Here's how the part is built. I have some questions about the finished solid (model axes, mm). A direction names the side the tool comes from. Give positions to 0.01 mm unless a question says otherwise; leave off trailing zeros. Loops run counter-clockwise (first coordinate to the right, second up) from the corner with the lowest first, then second, coordinate; pieces in that order, holes last. Notation, with made-up numbers: (-24, 22) - (-20, 22) arc R21 cw to (-20, 41) - close; hole circle Ø4 at (58.25, 12). An arc over 180 degrees is marked (long way). Use one line per item in the form item = value.
from build123d import *

# Parameters (mm, degrees)
F0_R     = 3.175
F1_DEPTH = 3.175


with BuildPart() as f1:
    # F0 (on Right) → F1 (new body)
    with BuildSketch(Plane.YZ):
        with BuildLine():
            Line((-11.176, 44.45), (-7.62, 0))
            ThreePointArc((-7.62, 0), (0, -7.62), (7.62, 0))
            Line((7.62, 0), (9.542272, 24.0284))
            ThreePointArc((9.542272, 24.0284), (11.848513, 29.596159), (17.416272, 31.9024))
            Line((17.416272, 31.9024), (63.5, 27.810218))
            Line((63.5, 27.810218), (115.700079, 31.9024))
            ThreePointArc((115.700079, 31.9024), (125.810106, 43.319551), (115.700079, 54.736701))
            Line((115.700079, 54.736701), (63.5, 61.099302))
            Line((63.5, 61.099302), (0, 55.626))
            ThreePointArc((0, 55.626), (-7.902625, 52.352625), (-11.176, 44.45))
        make_face()
        Circle(F0_R, mode=Mode.SUBTRACT)
        with Locations((0, 44.45)):
            Circle(F0_R, mode=Mode.SUBTRACT)
        with Locations((63.5, 44.45)):
            Circle(F0_R, mode=Mode.SUBTRACT)
        with Locations((99.822, 47.625)):
            Circle(F0_R, mode=Mode.SUBTRACT)
        with Locations((114.3, 44.45)):
            Circle(F0_R, mode=Mode.SUBTRACT)
    extrude(amount=F1_DEPTH)


solid = f1.part
(1) If we section it at D-D (y = 59): List the corners of the cut face in (x, z) for me (3 decimals).
Geometry says:
outline = (0, 28.21) - (3.175, 28.21) - (3.175, 60.711) - (0, 60.711) - close
(2) If we section it at A-A (y = 114.3): List the corners of the cut face in (x, z) for me (3 decimals), plus the area to 3 significant figures.
Geometry says:
outline = (0, 31.793) - (3.175, 31.793) - (3.175, 41.275) - (0, 41.275) - close; (0, 47.625) - (3.175, 47.625) - (3.175, 54.907) - (0, 54.907) - close
area = 53.2 mm²
(3) If I drill on probe 1 along Z at (x, y) = (1.1, 0) (3 decimals); probe 2 along Z at (x, y) = (2.7, 1.5); probe 3 along Y at (x, z) = (0.45, 48), over which ranges is the centre line in solid material (lowest first)?
Geometry says:
probe_1 = -7.62 to -3.175, 3.175 to 41.275, 47.625 to 55.626
probe_2 = -7.47 to -2.8, 2.8 to 41.65, 47.25 to 55.76
probe_3 = -10.6 to 96.67, 102.97 to 124.81
(4) For faces 1 (the flat face through (1.565, 40.136, 29.885)), 2 (the cylindrical face through (1.565, 1.707, 47.127)), which set-ups out of +Z, -Z, +X, -X, +Y, -Y let a thin tool reach every point of the face, with its end or its side?
Geometry says:
face_1 = -Z, +X, -X
face_2 = +X, -X
(5) If we section it at C-C (z = 20): List the corners of the cut face in (x, y) for me (3 decimals), plus the area to 3 significant figures.
Geometry says:
outline = (0, -9.22) - (3.175, -9.22) - (3.175, 9.22) - (0, 9.22) - close
area = 58.5 mm²
(6) Thinking about a two-plate mould opening in Z: for faces 3 (the cylindrical face through (1.565, 116.007, 47.127)), 4 (the cylindrical face through (1.565, 125.808, 43.086)), 5 (the flat face through (1.565, -9.423, 22.536)), which applies, pulls with the +Z half, pulls with the -Z half, needs draft (parallel to the pull), parting line crosses it, or undercut?
Geometry says:
face_3 = undercut
face_4 = parting line crosses it
face_5 = pulls with the -Z half
(7) For P1, Ø1.5, axis at x = 2, y = 84, coming from the -Z side; P2, Ø8.5, axis at y = 0, z = 0, coming from the -X side, each with a flat end and sliding along its axis, tell me the tip position at first contact or that it passes through.
Geometry says:
P1 = 29.36
P2 = 0
(8) If we section it at B-B (x = 2.35): List the corners of the cut face in (y, z) for me (3 decimals).
Geometry says:
outline = (-11.176, 44.45) - (-7.62, 0) arc R7.62 ccw to (7.62, 0) - (9.542, 24.028) arc R7.874 cw to (17.416, 31.902) - (63.5, 27.81) - (115.7, 31.902) arc R11.502 ccw to (115.7, 54.737) - (63.5, 61.099) - (0, 55.626) arc R11.176 ccw to start; hole circle Ø6.35 at (0, 0); hole circle Ø6.35 at (0, 44.45); hole circle Ø6.35 at (63.5, 44.45); hole circle Ø6.35 at (99.822, 47.625); hole circle Ø6.35 at (114.3, 44.45)
